Could you check a few things on this model? Use its own coordinates, in mm. A direction names the side the tool comes from. Coordinates: 2 decimals unless noted, no trailing zeros. Loops run counter-clockwise (first coordinate to the right, second up) from the corner with the lowest first, then second, coordinate; pieces in that order, holes last. Notation, with made-up numbers: (-12.75, 52) -> (19.25, 52) arc R27 cw to (19.25, 82) -> close; hole circle Ø5 at (58, 20). An arc over 180 degrees is marked (long way). One line per question, with ' | ' between items.
from build123d import *

# Parameters (mm, degrees)
EXTRUDE_1_DEPTH     = 2050
SHELL_1_T           = -4
CUT_EXTRUDE_1_REACH = 362
SKETCH_2_R          = 7
SKETCH_3_W          = 80
SKETCH_3_H          = 3.5
EXTRUDE_2_DEPTH     = 2050
FILLET_1_R          = 3
FILLET_2_R          = 6.5


with BuildPart() as part:
    # 草图1 → 凸台-拉伸1 (new body)
    with BuildSketch(Plane.XY):
        with BuildLine():
            Line((0, 0), (0, 43.672177815))
            ThreePointArc((0, 43.672177815), (-3.381974368, 51.168959573), (-11.240347346, 53.594956582))
            Line((-11.240347346, 53.594956582), (-351.240347346, 11.094956582))
            ThreePointArc((-351.240347346, 11.094956582), (-357.496781758, 7.790203447), (-360, 1.172177815))
            Line((-360, 1.172177815), (-360, -10))
            Line((-360, -10), (-300, -10))
            Line((-300, -10), (0, 0))
        make_face()
    extrude(amount=EXTRUDE_1_DEPTH)

    # 抽壳1
    shell_1_openings = [part.faces().sort_by_distance(p)[0] for p in [
        (-197.44558621, 13.389471059, 2050),
        (-330, -10, 1025),
        (-150, -5, 1025),
        (-197.44558621, 13.389471059, 0),
    ]]
    offset(amount=SHELL_1_T, openings=shell_1_openings, kind=Kind.INTERSECTION)

    # 草图2 → 切除-拉伸1 (cut, up to next)
    with BuildSketch(Plane(origin=(0, 0, 0), x_dir=(0, 0, -1), z_dir=(1, 0, 0)), mode=Mode.PRIVATE) as cut_extrude_1_sk1:
        with Locations((-2028, 28.672177815)):
            Circle(SKETCH_2_R)
    cut_extrude_1_tool1 = extrude(cut_extrude_1_sk1.sketch, amount=-CUT_EXTRUDE_1_REACH, mode=Mode.PRIVATE) & part.part
    add(cut_extrude_1_tool1.solids().sort_by_distance((0, 28.672178, 2028))[0], mode=Mode.SUBTRACT)
    # 草图2 → 切除-拉伸1 (cut, up to next)
    with BuildSketch(Plane(origin=(0, 0, 0), x_dir=(0, 0, -1), z_dir=(1, 0, 0)), mode=Mode.PRIVATE) as cut_extrude_1_sk2:
        with Locations((-1978, 28.672177815)):
            Circle(SKETCH_2_R)
    cut_extrude_1_tool2 = extrude(cut_extrude_1_sk2.sketch, amount=-CUT_EXTRUDE_1_REACH, mode=Mode.PRIVATE) & part.part
    add(cut_extrude_1_tool2.solids().sort_by_distance((0, 28.672178, 1978))[0], mode=Mode.SUBTRACT)
    # 草图2 → 切除-拉伸1 (cut, up to next)
    with BuildSketch(Plane(origin=(0, 0, 0), x_dir=(0, 0, -1), z_dir=(1, 0, 0)), mode=Mode.PRIVATE) as cut_extrude_1_sk3:
        with Locations((-1928, 28.672177815)):
            Circle(SKETCH_2_R)
    cut_extrude_1_tool3 = extrude(cut_extrude_1_sk3.sketch, amount=-CUT_EXTRUDE_1_REACH, mode=Mode.PRIVATE) & part.part
    add(cut_extrude_1_tool3.solids().sort_by_distance((0, 28.672178, 1928))[0], mode=Mode.SUBTRACT)
    # 草图2 → 切除-拉伸1 (cut, up to next)
    with BuildSketch(Plane(origin=(0, 0, 0), x_dir=(0, 0, -1), z_dir=(1, 0, 0)), mode=Mode.PRIVATE) as cut_extrude_1_sk4:
        with Locations((-122, 28.672177815)):
            Circle(SKETCH_2_R)
    cut_extrude_1_tool4 = extrude(cut_extrude_1_sk4.sketch, amount=-CUT_EXTRUDE_1_REACH, mode=Mode.PRIVATE) & part.part
    add(cut_extrude_1_tool4.solids().sort_by_distance((0, 28.672178, 122))[0], mode=Mode.SUBTRACT)
    # 草图2 → 切除-拉伸1 (cut, up to next)
    with BuildSketch(Plane(origin=(0, 0, 0), x_dir=(0, 0, -1), z_dir=(1, 0, 0)), mode=Mode.PRIVATE) as cut_extrude_1_sk5:
        with Locations((-72, 28.672177815)):
            Circle(SKETCH_2_R)
    cut_extrude_1_tool5 = extrude(cut_extrude_1_sk5.sketch, amount=-CUT_EXTRUDE_1_REACH, mode=Mode.PRIVATE) & part.part
    add(cut_extrude_1_tool5.solids().sort_by_distance((0, 28.672178, 72))[0], mode=Mode.SUBTRACT)
    # 草图2 → 切除-拉伸1 (cut, up to next)
    with BuildSketch(Plane(origin=(0, 0, 0), x_dir=(0, 0, -1), z_dir=(1, 0, 0)), mode=Mode.PRIVATE) as cut_extrude_1_sk6:
        with Locations((-22, 28.672177815)):
            Circle(SKETCH_2_R)
    cut_extrude_1_tool6 = extrude(cut_extrude_1_sk6.sketch, amount=-CUT_EXTRUDE_1_REACH, mode=Mode.PRIVATE) & part.part
    add(cut_extrude_1_tool6.solids().sort_by_distance((0, 28.672178, 22))[0], mode=Mode.SUBTRACT)
    # 草图2 → 切除-拉伸1 (cut, up to next)
    with BuildSketch(Plane(origin=(0, 0, 0), x_dir=(0, 0, -1), z_dir=(1, 0, 0)), mode=Mode.PRIVATE) as cut_extrude_1_sk7:
        with Locations((-1025, 28.672177815)):
            Circle(SKETCH_2_R)
    cut_extrude_1_tool7 = extrude(cut_extrude_1_sk7.sketch, amount=-CUT_EXTRUDE_1_REACH, mode=Mode.PRIVATE) & part.part
    add(cut_extrude_1_tool7.solids().sort_by_distance((0, 28.672178, 1025))[0], mode=Mode.SUBTRACT)
    # 草图2 → 切除-拉伸1 (cut, up to next)
    with BuildSketch(Plane(origin=(0, 0, 0), x_dir=(0, 0, -1), z_dir=(1, 0, 0)), mode=Mode.PRIVATE) as cut_extrude_1_sk8:
        with Locations((-1075, 28.672177815)):
            Circle(SKETCH_2_R)
    cut_extrude_1_tool8 = extrude(cut_extrude_1_sk8.sketch, amount=-CUT_EXTRUDE_1_REACH, mode=Mode.PRIVATE) & part.part
    add(cut_extrude_1_tool8.solids().sort_by_distance((0, 28.672178, 1075))[0], mode=Mode.SUBTRACT)
    # 草图2 → 切除-拉伸1 (cut, up to next)
    with BuildSketch(Plane(origin=(0, 0, 0), x_dir=(0, 0, -1), z_dir=(1, 0, 0)), mode=Mode.PRIVATE) as cut_extrude_1_sk9:
        with Locations((-975, 28.672177815)):
            Circle(SKETCH_2_R)
    cut_extrude_1_tool9 = extrude(cut_extrude_1_sk9.sketch, amount=-CUT_EXTRUDE_1_REACH, mode=Mode.PRIVATE) & part.part
    add(cut_extrude_1_tool9.solids().sort_by_distance((0, 28.672178, 975))[0], mode=Mode.SUBTRACT)

    # 草图3 → 凸台-拉伸2 (add)
    with BuildSketch(Plane.XY.offset(2050)):
        with Locations((-320, -8.25)):
            Rectangle(SKETCH_3_W, SKETCH_3_H)
    extrude(amount=-EXTRUDE_2_DEPTH)

    # 圆角1
    fillet_1_edges = [part.edges().sort_by_distance(p)[0] for p in [
        (-356, -6.5, 1025),
    ]]
    fillet(fillet_1_edges, radius=FILLET_1_R)

    # 圆角2
    fillet_2_edges = [part.edges().sort_by_distance(p)[0] for p in [
        (-360, -10, 1025),
    ]]
    fillet(fillet_2_edges, radius=FILLET_2_R)


solid = part.part
1) I need wall thicknesses on line 1 along Y through (x, z) = (-2, 2028); line 2 along Y through (x, z) = (-2.3, 1978); line 3 along X through (y, z) = (-5, 739). Which ranges of each line are inside material? Lowest first, please. Write a range as from..to.
Data:
line 1: -0.07..21.67, 35.67..49.67 | line 2: -0.08..21.67, 35.67..50.05 | line 3: -359.82..-355.6
2) I'm going to push flat-ended pins straight in: pin 1 Ø6 at (x, z) = (-122.5, 661) entering from -Y; pin 2 Ø1.8 at (y, z) = (-8, 562.5) entering from +X; pin 3 Ø8 at (x, y) = (-39, 42) entering from -Z; pin 4 Ø6 at (y, z) = (19, 1656.5) entering from +X. Where does each tip first touch, or does it pass through?
Data:
pin 1: y = 35.28 | pin 2: x = -280 | pin 3: through | pin 4: x = 0
3) If we section it at C-C on x = -185: Please give me the cut outline in (y, z) (3 decimals).
Data:
outline: (27.844, 0) -> (31.875, 0) -> (31.875, 2050) -> (27.844, 2050) -> close
4) We'd pull the mould along X, two halves only. Please class faces 3 (the face through (-178.364, 28.673, 1010.65)), 4 (the face through (-194, 27, 0)), 5 (the face through (0, 22, 1011)), 6 (the face through (-4, 21, 1011)): pulls with the +X half, pulls with the -X half, needs draft (parallel to the pull), parting line crosses it, or undercut.
Data:
face 3: undercut | face 4: needs draft | face 5: pulls with the +X half | face 6: undercut
5) If we section it at A-A on x = -310.5: Please give me the cut outline in (y, z), and give its area (3 significant figures).
Data:
outline: (-10, 0) -> (-6.5, 0) -> (-6.5, 2050) -> (-10, 2050) -> close; (12.16, 0) -> (16.19, 0) -> (16.19, 2050) -> (12.16, 2050) -> close | area: 15,400 mm²
6) If we section it at B-B on z = 604.5: Please give me the cut outline in (x, y).
Data:
outline: (-360, -3.5) arc R6.5 ccw to (-353.5, -10) -> (-280, -10) -> (-280, -6.5) -> (-353, -6.5) arc R3 cw to (-356, -3.5) -> (-356, 1.17) arc R6 cw to (-350.74, 7.13) -> (-10.74, 49.63) arc R6 cw to (-4, 43.67) -> (-4, -0.13) -> (0, 0) -> (0, 43.67) arc R10 ccw to (-11.24, 53.59) -> (-351.24, 11.09) arc R10 ccw to (-360, 1.17) -> close
7) On a 3-axis mill with a long thin cutter (end or side, diameter ignored), from which of +Z, -Z, +X, -X, +Y, -Y can I reach the whole of each face in a straight line? I mean faces 1 (the face through (-317, -6.5, 1039)), 2 (the face through (-317, -10, 1011)). Say none if no direction works.
Data:
face 1: +Z, -Z, +X | face 2: +Z, -Z, +X, -X, -Y
